Geometry check sheet. Reference: the model listing, model coordinates, mm. Face numbers are marked on the shaded views. A direction names the side the tool comes from. Give positions to 0.01 mm unless a question says otherwise; leave off trailing zeros. Write each loop counter-clockwise with the first axis right and the second up, starting at its lowest first coordinate (ties: lowest second). Pieces come first, ordered by that corner, then holes. Notation, with made-up numbers: (85.5, 70) -> (120.5, 70) arc R19 cw to (120.5, 83) -> close; hole circle Ø1 at (-38, 75). An arc over 180 degrees is marked (long way). One line per item, written item: value.
from build123d import *

# Parameters (mm, degrees)
F0_R     = 7.62
F1_DEPTH = 63.5
F0_R_2   = 34.925
F3_DEPTH = 6.35
F4_DEPTH = 73.66


# Not quite as in the source:
# - the program builds the solid bodies; features that only make, move or delete a surface that nothing else refers to are left out


with BuildPart() as f1:
    # F0 (on Top) → F1 (new body)
    with BuildSketch(Plane.XY):
        with BuildLine():
            ThreePointArc((19.6950692857, -10.2982945593), (11.6205, 0), (19.6950692857, 10.2982945593))
            ThreePointArc((19.6950692857, 10.2982945593), (15.0819932796, 16.3243408355), (8.7103855253, 20.447))
            ThreePointArc((8.7103855253, 20.447), (0, 13.335), (-8.7103855253, 20.447))
            ThreePointArc((-8.7103855253, 20.447), (-14.4936529558, 16.8488767874), (-18.9156521429, 11.668278751))
            ThreePointArc((-18.9156521429, 11.668278751), (-12.549310419, 7.3131076419), (-10.0965, 0))
            ThreePointArc((-10.0965, 0), (-12.549310419, -7.3131076419), (-18.9156521429, -11.668278751))
            ThreePointArc((-18.9156521429, -11.668278751), (-14.738135996, -16.6354432572), (-9.3037440003, -20.1839285714))
            ThreePointArc((-9.3037440003, -20.1839285714), (0, -12.7), (9.3037440003, -20.1839285714))
            ThreePointArc((9.3037440003, -20.1839285714), (15.3187542886, -16.102372249), (19.6950692857, -10.2982945593))
        make_face()
        Circle(F0_R, mode=Mode.SUBTRACT)
    extrude(amount=-F1_DEPTH)

    # F0 (on Top) → F3 (join)
    with BuildSketch(Plane.XY):
        Circle(F0_R_2)
        with BuildLine():
            ThreePointArc((8.7103855253, 20.447), (15.0819932796, 16.3243408355), (19.6950692857, 10.2982945593))
            ThreePointArc((19.6950692857, 10.2982945593), (28.7681937917, 8.3451803608), (32.8295, 0))
            ThreePointArc((32.8295, 0), (28.7681937917, -8.3451803608), (19.6950692857, -10.2982945593))
            ThreePointArc((19.6950692857, -10.2982945593), (15.3187542886, -16.102372249), (9.3037440003, -20.1839285714))
            ThreePointArc((9.3037440003, -20.1839285714), (9.4695244496, -21.198485656), (9.525, -22.225))
            ThreePointArc((9.525, -22.225), (-1.026514344, -31.6945244496), (-9.3037440003, -20.1839285714))
            ThreePointArc((-9.3037440003, -20.1839285714), (-14.738135996, -16.6354432572), (-18.9156521429, -11.668278751))
            ThreePointArc((-18.9156521429, -11.668278751), (-34.3535, 0), (-18.9156521429, 11.668278751))
            ThreePointArc((-18.9156521429, 11.668278751), (-14.4936529558, 16.8488767874), (-8.7103855253, 20.447))
            ThreePointArc((-8.7103855253, 20.447), (-0.8935246722, 31.0699824002), (8.89, 22.225))
            ThreePointArc((8.89, 22.225), (8.8449824002, 21.3314753278), (8.7103855253, 20.447))
        make_face(mode=Mode.SUBTRACT)
        with BuildLine():
            ThreePointArc((19.6950692857, -10.2982945593), (11.6205, 0), (19.6950692857, 10.2982945593))
            ThreePointArc((19.6950692857, 10.2982945593), (15.0819932796, 16.3243408355), (8.7103855253, 20.447))
            ThreePointArc((8.7103855253, 20.447), (0, 13.335), (-8.7103855253, 20.447))
            ThreePointArc((-8.7103855253, 20.447), (-14.4936529558, 16.8488767874), (-18.9156521429, 11.668278751))
            ThreePointArc((-18.9156521429, 11.668278751), (-12.549310419, 7.3131076419), (-10.0965, 0))
            ThreePointArc((-10.0965, 0), (-12.549310419, -7.3131076419), (-18.9156521429, -11.668278751))
            ThreePointArc((-18.9156521429, -11.668278751), (-14.738135996, -16.6354432572), (-9.3037440003, -20.1839285714))
            ThreePointArc((-9.3037440003, -20.1839285714), (0, -12.7), (9.3037440003, -20.1839285714))
            ThreePointArc((9.3037440003, -20.1839285714), (15.3187542886, -16.102372249), (19.6950692857, -10.2982945593))
        make_face()
        Circle(F0_R, mode=Mode.SUBTRACT)
        with BuildLine():
            ThreePointArc((-8.7103855253, 20.447), (0, 13.335), (8.7103855253, 20.447))
            ThreePointArc((8.7103855253, 20.447), (0, 22.225), (-8.7103855253, 20.447))
        make_face()
        with BuildLine():
            ThreePointArc((-8.7103855253, 20.447), (0, 22.225), (8.7103855253, 20.447))
            ThreePointArc((8.7103855253, 20.447), (8.8449824002, 21.3314753278), (8.89, 22.225))
            ThreePointArc((8.89, 22.225), (-0.8935246722, 31.0699824002), (-8.7103855253, 20.447))
        make_face()
        with BuildLine():
            ThreePointArc((19.6950692857, -10.2982945593), (21.5832520705, -5.30225), (22.225, 0))
            ThreePointArc((22.225, 0), (21.5832520705, 5.30225), (19.6950692857, 10.2982945593))
            ThreePointArc((19.6950692857, 10.2982945593), (11.6205, 0), (19.6950692857, -10.2982945593))
        make_face()
        with BuildLine():
            ThreePointArc((19.6950692857, 10.2982945593), (21.5832520705, 5.30225), (22.225, 0))
            ThreePointArc((22.225, 0), (21.5832520705, -5.30225), (19.6950692857, -10.2982945593))
            ThreePointArc((19.6950692857, -10.2982945593), (28.7681937917, -8.3451803608), (32.8295, 0))
            ThreePointArc((32.8295, 0), (28.7681937917, 8.3451803608), (19.6950692857, 10.2982945593))
        make_face()
        with BuildLine():
            ThreePointArc((-18.9156521429, -11.668278751), (-22.225, 0), (-18.9156521429, 11.668278751))
            ThreePointArc((-18.9156521429, 11.668278751), (-34.3535, 0), (-18.9156521429, -11.668278751))
        make_face()
        with BuildLine():
            ThreePointArc((-10.0965, 0), (-12.549310419, 7.3131076419), (-18.9156521429, 11.668278751))
            ThreePointArc((-18.9156521429, 11.668278751), (-22.225, 0), (-18.9156521429, -11.668278751))
            ThreePointArc((-18.9156521429, -11.668278751), (-12.549310419, -7.3131076419), (-10.0965, 0))
        make_face()
        with BuildLine():
            ThreePointArc((9.525, -22.225), (9.4695244496, -21.198485656), (9.3037440003, -20.1839285714))
            ThreePointArc((9.3037440003, -20.1839285714), (0, -22.225), (-9.3037440003, -20.1839285714))
            ThreePointArc((-9.3037440003, -20.1839285714), (-1.026514344, -31.6945244496), (9.525, -22.225))
        make_face()
        with BuildLine():
            ThreePointArc((-9.3037440003, -20.1839285714), (0, -22.225), (9.3037440003, -20.1839285714))
            ThreePointArc((9.3037440003, -20.1839285714), (0, -12.7), (-9.3037440003, -20.1839285714))
        make_face()
    extrude(amount=F3_DEPTH)

    # F0 (on Top) → F4 (join)
    with BuildSketch(Plane.XY):
        Circle(F0_R)
    extrude(amount=-F4_DEPTH)


solid = f1.part
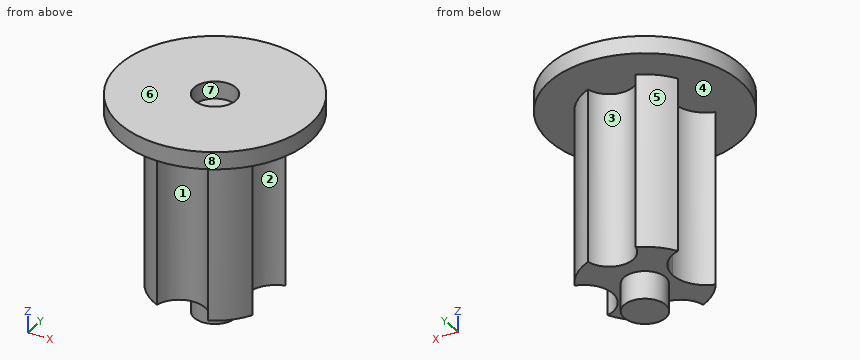
1) Scan lines: probe 1 along Y at (x, z) = (0, 4) (3 decimals); probe 2 along Z at (x, y) = (-19.5, -13); probe 3 along X at (y, z) = (-15, -51). Record each from-to range of solid material in increasing order.
Verdict:
probe 1: -34.925 to -7.62, 7.62 to 34.925
probe 2: 0 to 6.35
probe 3: -16.4 to -6.21, 6.21 to 16.4
2) Sectioned sample at C-C on y = 2. Record the cut outline in (x, z), plus the area to 3 significant figures.
Verdict:
outline: (-34.87, 0) -> (-10.26, 0) -> (-10.26, -63.5) -> (-7.35, -63.5) -> (-7.35, -73.66) -> (7.35, -73.66) -> (7.35, -63.5) -> (11.81, -63.5) -> (11.81, 0) -> (34.87, 0) -> (34.87, 6.35) -> (7.35, 6.35) -> (7.35, 0) -> (-7.35, 0) -> (-7.35, 6.35) -> (-34.87, 6.35) -> close
area: 1,900 mm^2
3) Sectioned sample at D-D on x = -13. Record the cut outline in (y, z).
Verdict:
outline: (-32.42, 0) -> (-18.03, 0) -> (-18.03, -63.5) -> (-7.87, -63.5) -> (-7.87, 0) -> (7.87, 0) -> (7.87, -63.5) -> (18.03, -63.5) -> (18.03, 0) -> (32.42, 0) -> (32.42, 6.35) -> (-32.42, 6.35) -> close
4) Depth check by flat-ended pin: pin 1 Ø1 at (x, z) = (11.5, -29.5) entering from -Y; pin 2 Ø2 at (x, y) = (24.5, -17.5) entering from -Z; pin 3 Ø4.5 at (x, y) = (3, -3) entering from +Z. Enter the tip coordinate at first touch or a pass-through.
Verdict:
pin 1: y = -19.31
pin 2: z = 0
pin 3: z = 0
5) Sectioned sample at A-A on x = 0. Record the cut outline in (y, z) (3 decimals), plus the area to 3 significant figures.
Verdict:
outline: (-34.925, 0) -> (-12.7, 0) -> (-12.7, -63.5) -> (-7.62, -63.5) -> (-7.62, -73.66) -> (7.62, -73.66) -> (7.62, -63.5) -> (13.335, -63.5) -> (13.335, 0) -> (34.925, 0) -> (34.925, 6.35) -> (7.62, 6.35) -> (7.62, 0) -> (-7.62, 0) -> (-7.62, 6.35) -> (-34.925, 6.35) -> close
area: 2,150 mm^2
6) Mould release check, pull along X, two halves, no side actions. Record for the marked faces 6, 7 and 8: released by +X, released by -X, zero draft, split by the parting line, or undercut.
Verdict:
face 6: zero draft
face 7: undercut
face 8: split by the parting line
7) Tool access check on the marked faces 1, 2, 3, 4 and 5. Record the directions out of +Z, -Z, +X, -X, +Y, -Y that give a thin tool (end or side, any length) a straight path to the whole face; none if there is none.
Verdict:
face 1: -Z, -Y
face 2: -Z, +X
face 3: -Z, +Y
face 4: -Z
face 5: -Z, -X, +Y
